The listing builds one solid part. Answer for the finished solid, in the listing's coordinates (mm). A direction names the side the tool comes from. Give positions to 0.01 mm unless a question says otherwise; leave off trailing zeros. Write each loop counter-clockwise with the first axis right and the second up, starting at its lowest first coordinate (ties: lowest second). Pieces come first, ordered by that corner, then holes. Notation, with made-up numbers: (71.5, 10.5) -> (129.5, 10.5) arc R27 ccw to (129.5, 44.5) -> close; hole circle Ø8 at (22, -39.5). An arc over 180 degrees is marked (long way). Put each result on its own line as item: value. Start each with the question number.
1) For a pull along Z with two mould halves and no side action, classify faces 5 (the flat face through (8, -10, 13)), 6 (the cylindrical face through (-30.44, 32.02, 25.51)), 7 (the cylindrical face through (-37.44, -11.48, 32.51)), 8 (the flat face through (-18, 32, 35.5)) as released by +Z, released by -Z, zero draft, split by the parting line, or undercut.
2) Find the intervals of material crossed by line 1 along Y through (x, z) = (-17, 16); line 2 along Y through (x, z) = (7, 6); line 3 along Z through (x, y) = (6, 1.5), in increasing order. Write a range as from..to.
3) A cutting plane is placed at C-C (y = 16). Write down the section's boundary in (x, z) (3 decimals).
4) A cutting plane is placed at B-B (z = 4). Write down the section's boundary in (x, y), then the cut area to 3 significant figures.
5) For faces 1 (the cylindrical face through (0.11, -0.74, 0.95)), 2 (the flat face through (0, 10, -0.5)), 3 (the flat face through (-12, 24, 0)), 4 (the flat face through (-26, -12, 13.58)), determine the directions among +Z, -Z, +X, -X, +Y, -Y from which every point of the face is accessible in a straight line to the end or side of a thin tool.
6) A cutting plane is placed at A-A (x = -17.5). Write down the section's boundary in (y, z), then the cut area to 3 significant figures.
7) A cutting plane is placed at D-D (x = -2.5). Write down the section's boundary in (y, z), then the cut area to 3 significant figures.
8) Flat-ended cylindrical pins translate along their axes: pin 1 Ø1.5 at (x, y) = (-4, -7.5) entering from -Z; pin 2 Ø1.5 at (y, z) = (3, 29) entering from -X; pin 3 Ø2.5 at (x, y) = (7, 9) entering from -Z. Find the tip coordinate at first contact, or state that the pin passes through.
from build123d import *

# Parameters (mm, degrees)
SKETCH1_W           = 23.83
SKETCH1_H           = 1
BOSS_EXTRUDE1_DEPTH = 20.5
SKETCH2_R           = 1.325
BOSS_EXTRUDE2_DEPTH = 13.75
BOSS_EXTRUDE4_DEPTH = 8
SKETCH5_W           = 21.919818374
SKETCH5_H           = 2.5
BOSS_EXTRUDE5_DEPTH = 40
SKETCH6_R           = 4.25
SKETCH6_R_2         = 1.05
CUT_EXTRUDE1_DEPTH  = 76.367433285
FILLET1_R           = 7
FILLET2_R           = 7
FILLET3_R           = 7
BOSS_EXTRUDE6_START = 41
BOSS_EXTRUDE6_DEPTH = 41


with BuildPart() as part:
    # Sketch1 → Boss-Extrude1 (new body)
    with BuildSketch(Plane(origin=(0, 0, 0), x_dir=(1, 0, 0), z_dir=(0, 1, 0))):
        Rectangle(SKETCH1_W, SKETCH1_H)
    extrude(amount=BOSS_EXTRUDE1_DEPTH)

    # Sketch2 → Boss-Extrude2 (add, symmetric)
    with BuildSketch(Plane(origin=(0, 10.25, 0), x_dir=(1, 0, 0), z_dir=(0, 1, 0))):
        with Locations(Location((-11.915, 0, 0), (0, 0, 270))):
            Circle(SKETCH2_R)
        with Locations(Location((11.915, 0, 0), (0, 0, 270))):
            Circle(SKETCH2_R)
    extrude(amount=BOSS_EXTRUDE2_DEPTH, both=True)

    # Sketch4 → Boss-Extrude4 (add, symmetric)
    with BuildSketch(Plane(origin=(0, 0, 0), x_dir=(0, 0, -1), z_dir=(1, 0, 0))):
        Polygon((-0.5, 16.852307022), (-0.5, 20.5), (-12.5, 33.25), (-35.5, 33.25), (-35.5, 30.75), (-13.580181626, 30.75), align=None)
        Polygon((-0.5, 0), (-0.5, 3.647692978), (-13.580181626, -10.25), (-35.5, -10.25), (-35.5, -12.75), (-12.5, -12.75), align=None)
    extrude(amount=BOSS_EXTRUDE4_DEPTH, both=True)

    # Sketch5 → Boss-Extrude5 (add)
    with BuildSketch(Plane.ZY.offset(8)):
        with Locations((24.540090813, 32)):
            Rectangle(SKETCH5_W, SKETCH5_H)
        with Locations((24.540090813, -11.5)):
            Rectangle(SKETCH5_W, SKETCH5_H)
    extrude(amount=BOSS_EXTRUDE5_DEPTH)

    # Sketch6 → Cut-Extrude1 (cut, through all)
    with BuildSketch(Plane(origin=(0, 33.25, 0), x_dir=(1, 0, 0), z_dir=(0, 1, 0))):
        with Locations(Location((-37.040090813, -24.540090813, 0), (0, 0, 270))):
            Circle(SKETCH6_R)
        with Locations(Location((-44.040090813, -24.540090813, 0), (0, 0, 270))):
            Circle(SKETCH6_R_2)
        with Locations(Location((-37.040090813, -17.540090813, 0), (0, 0, 270))):
            Circle(SKETCH6_R_2)
        with Locations(Location((-30.040090813, -24.540090813, 0), (0, 0, 270))):
            Circle(SKETCH6_R_2)
        with Locations(Location((-37.040090813, -31.540090813, 0), (0, 0, 270))):
            Circle(SKETCH6_R_2)
        with BuildLine():
            ThreePointArc((-48, -24.540090813), (-44.78991692, -16.790264706), (-37.040090813, -13.580181626))
            Line((-37.040090813, -13.580181626), (-48, -13.580181626))
            Line((-48, -13.580181626), (-48, -24.540090813))
        make_face()
        with BuildLine():
            ThreePointArc((-37.040090813, -35.5), (-44.78991692, -32.28991692), (-48, -24.540090813))
            Line((-48, -24.540090813), (-48, -35.5))
            Line((-48, -35.5), (-37.040090813, -35.5))
        make_face()
    extrude(amount=-CUT_EXTRUDE1_DEPTH, mode=Mode.SUBTRACT)

    # Fillet1
    # the kernel refuses this fillet: 7 mm, written as the material it adds along each edge
    with BuildSketch(Plane(origin=(-8, -12.75, 13.580181626), x_dir=(-1, 0, 0), z_dir=(0, 1, 0))) as fillet1_piece_1_section:
        with BuildLine():
            CenterArc((FILLET1_R, -FILLET1_R), FILLET1_R, 90, 90)
            Line((0, -FILLET1_R), (0, 0))
            Line((0, 0), (FILLET1_R, 0))
        make_face()
    fillet1_piece_1 = extrude(amount=2.5, mode=Mode.PRIVATE)
    fillet1_piece_1 = split(fillet1_piece_1, bisect_by=Plane(origin=(-10.020174451, -12.153760937, 11.938833823), z_dir=(0, 0.6853646990049913, 0.7281999926928027)), keep=Keep.TOP, mode=Mode.PRIVATE)
    fillet1_piece_1 = split(fillet1_piece_1, bisect_by=Plane(origin=(-10.020174451, -10.440349189, 13.759333804), z_dir=(0, -0.685364699004991, -0.7281999926928029)), keep=Keep.TOP, mode=Mode.PRIVATE)
    add(fillet1_piece_1)
    with BuildSketch(Plane(origin=(-8, -12.75, 13.580181626), x_dir=(-1, 0, 0), z_dir=(0, 1, 0))) as fillet1_piece_2_section:
        with BuildLine():
            CenterArc((FILLET1_R, -FILLET1_R), FILLET1_R, 90, 90)
            Line((0, -FILLET1_R), (0, 0))
            Line((0, 0), (FILLET1_R, 0))
        make_face()
    fillet1_piece_2 = extrude(amount=20, mode=Mode.PRIVATE)
    fillet1_piece_2 = split(fillet1_piece_2, bisect_by=Plane(origin=(-8.816209607, -9.698679662, 9.628169093), z_dir=(0, 0.6853646990049913, 0.7281999926928027)), keep=Keep.TOP, mode=Mode.PRIVATE)
    fillet1_piece_2 = split(fillet1_piece_2, bisect_by=Plane(origin=(-8.816209607, -10.25, 10.809130305), z_dir=(0, 1, 0)), keep=Keep.TOP, mode=Mode.PRIVATE)
    fillet1_piece_2 = split(fillet1_piece_2, bisect_by=Plane(origin=(-8.816209607, -7.985267914, 11.448669075), z_dir=(0, -0.685364699004991, -0.7281999926928029)), keep=Keep.TOP, mode=Mode.PRIVATE)
    add(fillet1_piece_2)
    with BuildSketch(Plane(origin=(-8, 33.25, 13.580181626), x_dir=(0, 0, -1), z_dir=(0, -1, 0))) as fillet1_piece_3_section:
        with BuildLine():
            CenterArc((FILLET1_R, -FILLET1_R), FILLET1_R, 90, 90)
            Line((0, -FILLET1_R), (0, 0))
            Line((0, 0), (FILLET1_R, 0))
        make_face()
    fillet1_piece_3 = extrude(amount=2.5, mode=Mode.PRIVATE)
    fillet1_piece_3 = split(fillet1_piece_3, bisect_by=Plane(origin=(-10.020174451, 32.653760936, 11.938833823), z_dir=(0, -0.6853646990049912, 0.7281999926928028)), keep=Keep.TOP, mode=Mode.PRIVATE)
    fillet1_piece_3 = split(fillet1_piece_3, bisect_by=Plane(origin=(-10.020174451, 30.940349189, 13.759333804), z_dir=(0, 0.6853646990049909, -0.7281999926928031)), keep=Keep.TOP, mode=Mode.PRIVATE)
    add(fillet1_piece_3)
    with BuildSketch(Plane(origin=(-8, 33.25, 13.580181626), x_dir=(0, 0, -1), z_dir=(0, -1, 0))) as fillet1_piece_4_section:
        with BuildLine():
            CenterArc((FILLET1_R, -FILLET1_R), FILLET1_R, 90, 90)
            Line((0, -FILLET1_R), (0, 0))
            Line((0, 0), (FILLET1_R, 0))
        make_face()
    fillet1_piece_4 = extrude(amount=20, mode=Mode.PRIVATE)
    fillet1_piece_4 = split(fillet1_piece_4, bisect_by=Plane(origin=(-8.816209616, 30.198679665, 9.628169097), z_dir=(0, -0.6853646990049912, 0.7281999926928028)), keep=Keep.TOP, mode=Mode.PRIVATE)
    fillet1_piece_4 = split(fillet1_piece_4, bisect_by=Plane(origin=(-8.816209616, 28.485267918, 11.448669078), z_dir=(0, 0.6853646990049909, -0.7281999926928031)), keep=Keep.TOP, mode=Mode.PRIVATE)
    fillet1_piece_4 = split(fillet1_piece_4, bisect_by=Plane(origin=(-8.816209616, 30.75, 10.809130308), z_dir=(0, -1, 0)), keep=Keep.TOP, mode=Mode.PRIVATE)
    add(fillet1_piece_4)
    # the kernel refuses this fillet: 7 mm, written as the material it takes off along each edge
    with BuildSketch(Plane(origin=(8, 7.25, 35.5), x_dir=(0, 0, -1), z_dir=(0, -1, 0))) as fillet1_2_piece_1:
        with BuildLine():
            CenterArc((FILLET1_R, -FILLET1_R), FILLET1_R, 90, 90)
            Line((0, -FILLET1_R), (0, 0))
            Line((0, 0), (FILLET1_R, 0))
        make_face()
    extrude(amount=37.5, mode=Mode.SUBTRACT)
    with BuildSketch(Plane(origin=(8, 50.75, 35.5), x_dir=(-1, 0, 0), z_dir=(0, -1, 0))) as fillet1_2_piece_2:
        with BuildLine():
            CenterArc((FILLET1_R, FILLET1_R), FILLET1_R, 180, 90)
            Line((0, FILLET1_R), (0, 0))
            Line((0, 0), (FILLET1_R, 0))
        make_face()
    extrude(amount=37.5, mode=Mode.SUBTRACT)

    # Fillet2
    fillet2_edges = [part.edges().sort_by_distance(p)[0] for p in [
        (0, 16.852307022, 0.5),
        (0, 3.647692978, 0.5),
    ]]
    fillet(fillet2_edges, radius=FILLET2_R)

    # Fillet3
    # the kernel refuses this fillet: 7 mm, written as the material it adds along each edge
    with BuildSketch(Plane(origin=(-8, 20.5, 0.5), x_dir=(0, 0.7281999926925888, 0.6853646990052185), z_dir=(1, 0, 0))) as fillet3_piece_1:
        with BuildLine():
            CenterArc((2.423417163, -7), FILLET3_R, 90, 26.366519243)
            Line((-0.685364699, -0.728199993), (0, 0))
            Line((0, 0), (2.423417163, 0))
        make_face()
    extrude(amount=16)
    with BuildSketch(Plane(origin=(8, 0, 0.5), x_dir=(0, 0, -1), z_dir=(-1, 0, 0))) as fillet3_piece_2:
        with BuildLine():
            CenterArc((3.436475374, 6.562285254), FILLET3_R, 223.264295411, 26.366519243)
            Line((-1.660924575, 1.764732361), (0, 0))
            Line((0, 0), (1, 0))
        make_face()
    extrude(amount=16)

    # Sketch8 → Boss-Extrude6 (add)
    with BuildSketch(Plane(origin=(0, -10.25, 0), x_dir=(1, 0, 0), z_dir=(0, 1, 0)).offset(BOSS_EXTRUDE6_START)):
        with BuildLine():
            ThreePointArc((1, -35.5), (5.949747468, -33.449747468), (8, -28.5))
            Line((8, -28.5), (5, -28.5))
            ThreePointArc((5, -28.5), (3.422054899, -30.922054899), (1, -32.5))
            Line((1, -32.5), (1, -35.5))
        make_face()
    extrude(amount=-BOSS_EXTRUDE6_DEPTH)


solid = part.part
Reply:
1. face 5: zero draft
1. face 6: undercut
1. face 7: undercut
1. face 8: released by +Z
2. line 1: y = -12.75..-10.25, 30.75..33.25
2. line 2: y = -5.84..-2.2, 22.7..26.34
2. line 3: z = -0.5..2.52, 28.5..33.4
3. outline: (-10.688, -0.5) -> (10.688, -0.5) arc R1.325 ccw (long way) to (10.688, 0.5) -> (8, 0.5) -> (8, 0.77) -> (-8, 0.77) -> (-8, 0.5) -> (-10.688, 0.5) arc R1.325 ccw (long way) to start; (1, 32.5) arc R7 cw to (5, 28.5) -> (8, 28.5) arc R7 ccw to (1, 35.5) -> close
4. outline: (-8, -3.72) -> (8, -3.72) -> (8, -0.07) -> (-8, -0.07) -> close; (-8, 20.57) -> (8, 20.57) -> (8, 24.22) -> (-8, 24.22) -> close
4. area: 117 mm2
5. face 1: -Z, -Y
5. face 2: -Z, +Y, -Y
5. face 3: +Z, -Z, +X, -X, +Y
5. face 4: -Z, -X, +Y, -Y
6. outline: (-12.75, 13.58) -> (-10.25, 13.58) -> (-10.25, 35.5) -> (-12.75, 35.5) -> close; (30.75, 13.58) -> (33.25, 13.58) -> (33.25, 35.5) -> (30.75, 35.5) -> close
6. area: 110 mm2
7. outline: (-12.75, 12.5) -> (-1.76, 2.16) arc R7 cw to (0, -0.5) -> (20.5, -0.5) arc R7 cw to (22.26, 2.16) -> (33.25, 12.5) -> (33.25, 35.5) -> (30.75, 35.5) -> (30.75, 13.58) -> (18.87, 2.4) arc R7 cw to (14.08, 0.5) -> (6.42, 0.5) arc R7 cw to (1.63, 2.4) -> (-10.25, 13.58) -> (-10.25, 35.5) -> (-12.75, 35.5) -> close
7. area: 227 mm2
8. pin 1: stops at z = 6.85
8. pin 2: stops at x = 4.37
8. pin 3: stops at z = -0.5
